```python
from build123d import *

# Parameters (mm, degrees)
SKETCH1_W           = 200
SKETCH1_H           = 100
BOSS_EXTRUDE1_DEPTH = 5
SKETCH2_R           = 1.75
CUT_EXTRUDE1_DEPTH  = 224.662692463
SKETCH4_R           = 1.75
CUT_EXTRUDE2_DEPTH  = 224.662692463
SKETCH6_W           = 50
SKETCH6_H           = 25
SKETCH6_W_2         = 27
SKETCH6_H_2         = 27
CUT_EXTRUDE4_DEPTH  = 224.662692463
SKETCH7_W           = 35
SKETCH7_H           = 50
SKETCH7_R           = 1.75
CUT_EXTRUDE5_DEPTH  = 224.662692463


with BuildPart() as part:
    # Sketch1 → Boss-Extrude1 (new body)
    with BuildSketch(Plane(origin=(0, 0, 0), x_dir=(1, 0, 0), z_dir=(0, 1, 0))):
        with Locations((100, 50)):
            Rectangle(SKETCH1_W, SKETCH1_H)
    extrude(amount=BOSS_EXTRUDE1_DEPTH)

    # Sketch2 → Cut-Extrude1 (cut, through all)
    with BuildSketch(Plane(origin=(0, 5, 0), x_dir=(1, 0, 0), z_dir=(0, 1, 0))):
        with Locations(Location((170, 60, 0), (0, 0, 270))):
            Circle(SKETCH2_R)
        with Locations(Location((170, 40, 0), (0, 0, 270))):
            Circle(SKETCH2_R)
        with Locations(Location((30, 40, 0), (0, 0, 270))):
            Circle(SKETCH2_R)
        with Locations(Location((30, 60, 0), (0, 0, 90))):
            Circle(SKETCH2_R)
        with Locations(Location((155, 40, 0), (0, 0, 270))):
            Circle(SKETCH2_R)
        with Locations(Location((155, 60, 0), (0, 0, 270))):
            Circle(SKETCH2_R)
        with Locations(Location((45, 60, 0), (0, 0, 270))):
            Circle(SKETCH2_R)
        with Locations(Location((45, 40, 0), (0, 0, 90))):
            Circle(SKETCH2_R)
    extrude(amount=-CUT_EXTRUDE1_DEPTH, mode=Mode.SUBTRACT)

    # Sketch4 → Cut-Extrude2 (cut, through all)
    with BuildSketch(Plane(origin=(0, 5, 0), x_dir=(1, 0, 0), z_dir=(0, 1, 0))):
        with Locations(Location((155, 50, 0), (0, 0, 270))):
            Circle(SKETCH4_R)
        with Locations(Location((45, 50, 0), (0, 0, 270))):
            Circle(SKETCH4_R)
    extrude(amount=-CUT_EXTRUDE2_DEPTH, mode=Mode.SUBTRACT)

    # Sketch6 → Cut-Extrude4 (cut, through all)
    with BuildSketch(Plane(origin=(0, 5, 0), x_dir=(1, 0, 0), z_dir=(0, 1, 0))):
        with Locations((25, 12.5)):
            Rectangle(SKETCH6_W, SKETCH6_H)
        with Locations((25, 87.5)):
            Rectangle(SKETCH6_W, SKETCH6_H)
        with Locations((82.5, 67.5)):
            Rectangle(SKETCH6_W_2, SKETCH6_H_2)
        with Locations((117.5, 67.5)):
            Rectangle(SKETCH6_W_2, SKETCH6_H_2)
        with Locations((82.5, 32.5)):
            Rectangle(SKETCH6_W_2, SKETCH6_H_2)
        with Locations((117.5, 32.5)):
            Rectangle(SKETCH6_W_2, SKETCH6_H_2)
        with Locations((175, 87.5)):
            Rectangle(SKETCH6_W, SKETCH6_H)
        with Locations((175, 12.5)):
            Rectangle(SKETCH6_W, SKETCH6_H)
    extrude(amount=-CUT_EXTRUDE4_DEPTH, mode=Mode.SUBTRACT)

    # Sketch7 → Cut-Extrude5 (cut, through all)
    # profile 1 of 2: a face of its own
    with BuildSketch(Plane(origin=(0, 5, 0), x_dir=(1, 0, 0), z_dir=(0, 1, 0))):
        with Locations((182.5, 50)):
            Rectangle(SKETCH7_W, SKETCH7_H)
        with Locations((170, 40)):
            Circle(SKETCH7_R, mode=Mode.SUBTRACT)
        with Locations((170, 60)):
            Circle(SKETCH7_R, mode=Mode.SUBTRACT)
    # profile 2 of 2: a face of its own
    with BuildSketch(Plane(origin=(0, 5, 0), x_dir=(1, 0, 0), z_dir=(0, 1, 0))):
        with Locations((17.5, 50)):
            Rectangle(SKETCH7_W, SKETCH7_H)
        with Locations((30, 40)):
            Circle(SKETCH7_R, mode=Mode.SUBTRACT)
        with Locations((30, 60)):
            Circle(SKETCH7_R, mode=Mode.SUBTRACT)
    extrude(amount=-CUT_EXTRUDE5_DEPTH, mode=Mode.SUBTRACT)


solid = part.part
```
Verification items for the finished model (mm, model axes). A direction names the side the tool comes from. Round coordinates to 2 decimals unless told otherwise and drop trailing zeros. Order: outer loops, then holes, each group sorted by start corner. A loop starts at its lowest first (then second) coordinate and runs counter-clockwise, first axis right, second up. Notation, with made-up numbers: (20, 42.25) - (24, 42.25) arc R21 ccw to (24, 61.25) - close; hole circle Ø8 at (43, 4). An arc over 180 degrees is marked (long way). Use CSV: the item, a comma, the result in double quotes.
(1) Section check B-B on z = -31.5. Record the boundary of the cut face in (x, y), and give its area (3 significant figures).
Entries:
outline,"(35, 0) - (69, 0) - (69, 5) - (35, 5) - close; (96, 0) - (104, 0) - (104, 5) - (96, 5) - close; (131, 0) - (165, 0) - (165, 5) - (131, 5) - close"
area,"380 mm^2"
(2) Access from +Z, -Z, +X, -X, +Y, -Y to the whole of each face (thin tool, end or side, straight path). Record for faces 4 (the face through (50, 3, -87)), 5 (the face through (42, 3, -25)), 6 (the face through (69, 3, -67)).
Entries:
face 4,"-Z, -X, +Y, -Y"
face 5,"+Z, -X, +Y, -Y"
face 6,"+Y, -Y"
(3) Section check A-A on x = 45. Record the boundary of the cut face in (y, z), and give its area (4 significant figures).
Entries:
outline,"(0, -75) - (5, -75) - (5, -61.75) - (0, -61.75) - close; (0, -58.25) - (5, -58.25) - (5, -51.75) - (0, -51.75) - close; (0, -48.25) - (5, -48.25) - (5, -41.75) - (0, -41.75) - close; (0, -38.25) - (5, -38.25) - (5, -25) - (0, -25) - close"
area,"197.5 mm^2"
(4) Gauge pin test, flat ends, axial feed: pin 1 Ø2.5 at (y, z) = (2.5, -84.5) entering from -X; pin 2 Ø2.5 at (x, y) = (44, 3) entering from -Z; pin 3 Ø1.5 at (y, z) = (3, -87) entering from +X. Record the tip position at first contact, or that the pin passes through.
Entries:
pin 1,"x = 50"
pin 2,"z = -75"
pin 3,"x = 150"
(5) Section check D-D on x = 72.5. Record the boundary of the cut face in (y, z).
Entries:
outline,"(0, -100) - (5, -100) - (5, -81) - (0, -81) - close; (0, -54) - (5, -54) - (5, -46) - (0, -46) - close; (0, -19) - (5, -19) - (5, 0) - (0, 0) - close"
(6) Section check C-C on y = 3.9. State how many separate pieces and enclosed holes the cut face has, and give its area (3 significant figures).
Entries:
separate pieces,"1"
enclosed holes,"10"
area,"8,530 mm^2"
(7) Mould release check, pull along Z, two halves, no side actions. Record for faces 1 (the face through (157, 3, -25)), 2 (the face through (99, 2, -100)), 3 (the face through (46.55, 2.54, -40.81)): released by +Z, released by -Z, zero draft, split by the parting line, or undercut.
Entries:
face 1,"released by +Z"
face 2,"released by -Z"
face 3,"undercut"
(8) Thickness scan on probe 1 along X at (y, z) = (1.9, -43); probe 2 along X at (y, z) = (3.75, -79.5); probe 3 along X at (y, z) = (2.6, -40). Record the ranges inside material, lowest first. Write a range as from..to.
Entries:
probe 1,"35..69, 96..104, 131..165"
probe 2,"50..69, 96..104, 131..150"
probe 3,"35..43.25, 46.75..69, 96..104, 131..153.25, 156.75..165"
